The figure shows three views and two pictorial views of one solid part (mm, origin at its lowest corner). Answer the questions. Round coordinates to 2 decimals unless told otherwise and drop trailing zeros. Write each loop counter-clockwise with the first axis right and the second up, starting at its lowest first coordinate (ties: lowest second). Pieces come first, ordered by that corner, then holes.
Item 1: Each of these flat-tipped pins is pushed along its axis until it touches: pin 1 (4 mm diameter, centred on x = 76, y = 5.5, fed in from +Z); pin 2 (2 mm diameter, centred on x = 18.75, z = 2, fed in from -Y). Where does it stop, or does it pass through?
Item 2: Find section D-D on x = 93. Give the vertices of the cut face in (y, z).
Item 3: For a pull along X with two mould halves and no side action, classify the marked faces 1, 2 and 3 as +X half, -X half, draft (parallel to the pull), parting line (faces both ways), or undercut.
Item 4: Find section B-B on z = 5.5. Give the vertices of the cut face in (x, y), then the cut area to 3 significant figures.
Item 5: Find section A-A on y = 9.25. Give the vertices of the cut face in (x, z), then the cut area to 4 significant figures.
Item 6: Find the intervals of material crossed by probe 1 along X at (y, z) = (1.9, 2); probe 2 along Y at (x, z) = (92, 8.25); probe 3 along X at (y, z) = (1.75, 4.75), in increasing order.
Item 7: Find section C-C on x = 9.25. Give the vertices of the cut face in (y, z), then the cut area to 3 significant figures.
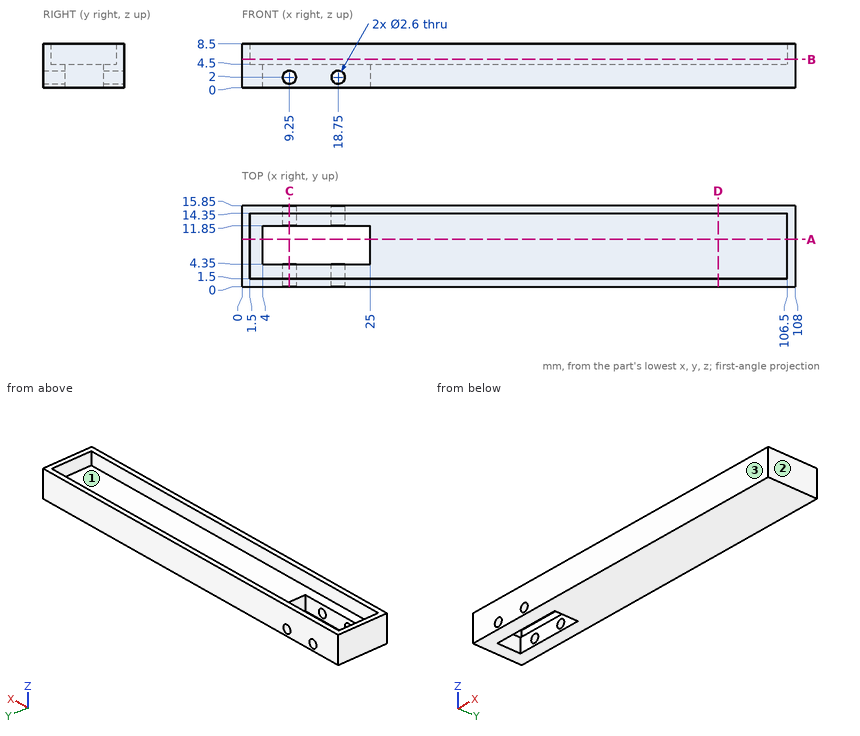
Check values:
1. pin 1: stops at z = 4.5
1. pin 2: passes through
2. outline: (0, 0) - (15.85, 0) - (15.85, 8.5) - (14.35, 8.5) - (14.35, 4.5) - (1.5, 4.5) - (1.5, 8.5) - (0, 8.5) - close
3. face 1: undercut
3. face 2: +X half
3. face 3: draft
4. outline: (0, 0) - (108, 0) - (108, 15.85) - (0, 15.85) - close; hole (1.5, 1.5) - (106.5, 1.5) - (106.5, 14.35) - (1.5, 14.35) - close
4. area: 363 mm2
5. outline: (0, 0) - (4, 0) - (4, 4.5) - (1.5, 4.5) - (1.5, 8.5) - (0, 8.5) - close; (25, 0) - (108, 0) - (108, 8.5) - (106.5, 8.5) - (106.5, 4.5) - (25, 4.5) - close
5. area: 403.5 mm2
6. probe 1: x = 0 to 7.95, 10.55 to 17.45, 20.05 to 108
6. probe 2: y = 0 to 1.5, 14.35 to 15.85
6. probe 3: x = 0 to 1.5, 106.5 to 108
7. outline: (0, 0) - (4.35, 0) - (4.35, 0.7) - (0, 0.7) - close; (0, 3.3) - (4.35, 3.3) - (4.35, 4.5) - (1.5, 4.5) - (1.5, 8.5) - (0, 8.5) - close; (11.85, 0) - (15.85, 0) - (15.85, 0.7) - (11.85, 0.7) - close; (11.85, 3.3) - (15.85, 3.3) - (15.85, 8.5) - (14.35, 8.5) - (14.35, 4.5) - (11.85, 4.5) - close
7. area: 27.9 mm2
